from build123d import *

# Parameters (mm, degrees)
SKETCH1_R               = 28.5
SKETCH1_R_2             = 14
BOSS_EXTRUDE1_DEPTH     = 7
SKETCH1_4_R             = 14
SKETCH1_4_R_2           = 3
BOSS_EXTRUDE2_DEPTH     = 25
SKETCH3_R               = 2.5
CUT_EXTRUDE1_DEPTH      = 1
CUT_EXTRUDE1_DEPTH_BACK = 26


with BuildPart() as part:
    # Sketch1 → Boss-Extrude1 (new body)
    with BuildSketch(Plane(origin=(0, 0, 0), x_dir=(0, 0, -1), z_dir=(1, 0, 0))):
        Circle(SKETCH1_R)
        Circle(SKETCH1_R_2, mode=Mode.SUBTRACT)
    extrude(amount=BOSS_EXTRUDE1_DEPTH)

    # Sketch1<4> → Boss-Extrude2 (add)
    with BuildSketch(Plane(origin=(0, 0, 0), x_dir=(0, 0, -1), z_dir=(1, 0, 0))):
        Circle(SKETCH1_4_R)
        Circle(SKETCH1_4_R_2, mode=Mode.SUBTRACT)
    extrude(amount=BOSS_EXTRUDE2_DEPTH)

    # Sketch3 → Cut-Extrude1 (cut, two sides)
    with BuildSketch(Plane.ZY) as cut_extrude1_sk:
        with Locations((19.055020887, -14.259950175)):
            Circle(SKETCH3_R)
        with Locations((11.9, -20.61140461)):
            Circle(SKETCH3_R)
        with Locations((2.52784293, -22.534415058)):
            Circle(SKETCH3_R)
        with Locations((-6.550188406, -19.513712423)):
            Circle(SKETCH3_R)
        with Locations((-12.901642841, -12.358691536)):
            Circle(SKETCH3_R)
        with Locations((-14.824653289, -2.986534466)):
            Circle(SKETCH3_R)
        with Locations((-11.803950653, 6.09149687)):
            Circle(SKETCH3_R)
        with Locations((-4.648929766, 12.442951305)):
            Circle(SKETCH3_R)
        with Locations((4.723227304, 14.365961753)):
            Circle(SKETCH3_R)
        with Locations((13.801258639, 11.345259118)):
            Circle(SKETCH3_R)
        with Locations((20.152713074, 4.19023823)):
            Circle(SKETCH3_R)
        with Locations((22.075723522, -5.18191884)):
            Circle(SKETCH3_R)
    extrude(amount=CUT_EXTRUDE1_DEPTH, mode=Mode.SUBTRACT)
    extrude(cut_extrude1_sk.sketch, amount=-CUT_EXTRUDE1_DEPTH_BACK, mode=Mode.SUBTRACT)


solid = part.part
Geometry: final body of the model. Coordinates: model frame, mm. A direction names the side the tool comes from. Give positions to 0.01 mm unless a question says otherwise; leave off trailing zeros. Order: outer loops, then holes, each group sorted by start corner. A loop starts at its lowest first (then second) coordinate and runs counter-clockwise, first axis right, second up. Notation, with made-up numbers: (-1.5, 29) - (46.5, 29) arc R10 ccw to (46.5, 40) - close; hole circle Ø1 at (84.5, 20). An arc over 180 degrees is marked (long way). Use CSV: the item, a comma, the result in double quotes.
1. Mould query, pull axis Z, two halves, no side actions, for faces 1 (the face through (15.87, -10.21, 9.58)), 2 (the face through (9.547, 11.925, 4.181)), 3 (the face through (3.45, 3.23, 22.46)), 4 (the face through (25, 0.2, 3.3)). Classes: +Z half, -Z half, draft (parallel to the pull), parting line (faces both ways), or undercut.
Answers below:
face 1,"parting line"
face 2,"undercut"
face 3,"undercut"
face 4,"draft"
2. Access query for faces 5 (the face through (3.451, -10.916, -26.327)), 6 (the face through (7, 7, 13)), 7 (the face through (16, 14, 0)). Directions: +Z, -Z, +X, -X, +Y, -Y. A direction counts if a zero-diameter tool reaches every point of the face in a straight line with its end or side. Return the directions, or none.
Answers below:
face 5,"+X, -X"
face 6,"+X"
face 7,"+X, +Y"
3. Section query D-D (y = 1). Output: boundary loops of the cut face in (x, z).
Answers below:
outline,"(0, -28.48) - (7, -28.48) - (7, -13.96) - (25, -13.96) - (25, -2.83) - (0, -2.83) - close; (0, 2.83) - (25, 2.83) - (25, 13.96) - (7, 13.96) - (7, 28.48) - (0, 28.48) - close"
4. Section query C-C (z = 1.5). Output: boundary loops of the cut face in (x, y).
Answers below:
outline,"(0, -28.46) - (7, -28.46) - (7, -24.81) - (0, -24.81) - close; (0, -20.26) - (7, -20.26) - (7, -13.92) - (25, -13.92) - (25, -2.6) - (0, -2.6) - close; (0, 2.6) - (25, 2.6) - (25, 13.92) - (7, 13.92) - (7, 28.46) - (0, 28.46) - close"
5. Material intervals for line 1 along Z through (x, y) = (3, -14.5); line 2 along Y through (x, z) = (2.25, 19); line 3 along X through (y, z) = (-22, 6), sorted ascending. Write a range as from..to.
Answers below:
line 1,"-24.54..-14.19, -11.61..16.57, 21.54..24.54"
line 2,"-21.24..-16.76, -11.76..1.97, 6.41..21.24"
line 3,"0..7"
6. Section query A-A (y = 16). Output: boundary loops of the cut face in (x, z).
Answers below:
outline,"(0, -23.58) - (7, -23.58) - (7, 2.83) - (0, 2.83) - close; (0, 6.62) - (7, 6.62) - (7, 23.58) - (0, 23.58) - close"
7. Section query B-B (x = 13.5). Output: boundary loops of the cut face in (y, z).
Answers below:
outline,"(-4.83, -13.14) arc R2.5 cw to (-0.63, -13.99) arc R14 ccw to (4.14, -13.37) arc R2.5 cw (long way) to (8.5, -11.13) arc R14 ccw to (12.06, -7.12) arc R2.5 cw (long way) to (13.77, -2.53) arc R14 ccw to (13.81, 2.29) arc R2.5 cw to (12.47, 6.36) arc R14 ccw (long way) to start; hole circle Ø6 at (0, 0)"
8. Contact query for flat-ended pins moving along their axis: pin 1 (6 mm diameter, centred on y = 11.35, z = 13.8, fed in from +X); pin 2 (12 mm diameter, centred on x = 11.5, z = 3.5, fed in from -Y); pin 3 (6 mm diameter, centred on x = 8, y = -22.5, fed in from +Z). Output: stop coordinate, or through.
Answers below:
pin 1,"x = 7"
pin 2,"y = -28.5"
pin 3,"z = 20.62"
